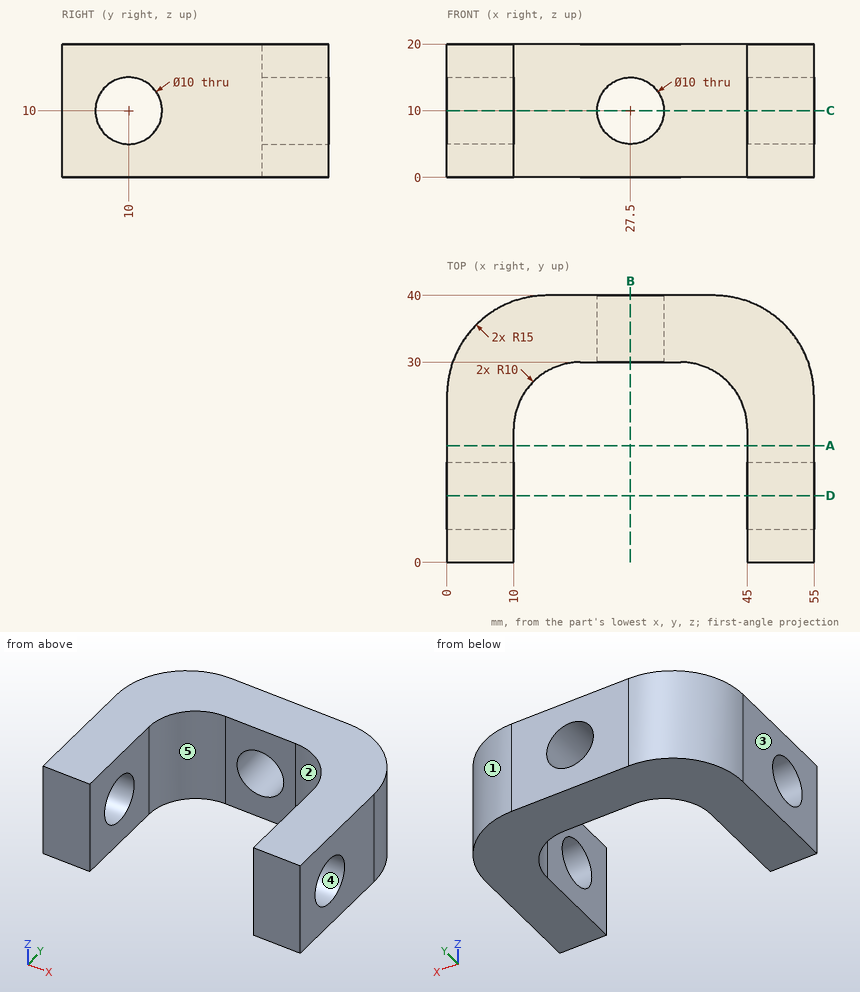
Study the drawing (mm; zero at the part's minimum x, y, z) and answer. A direction names the side the tool comes from. Give positions to 0.01 mm unless a question says otherwise; leave off trailing zeros. Write each loop counter-clockwise with the first axis right and the second up, starting at its lowest first coordinate (ties: lowest second). Pieces come first, ordered by that corner, then holes. Notation, with made-up numbers: (-1.75, 0.25) - (55.25, 0.25) arc R8 cw to (55.25, 15.25) - close; hole circle Ø6 at (33.25, 23.5). An arc over 180 degrees is marked (long way). One line per question, with ' | ' between items. Start each with the question number.
1. Determine the mould class of the marked faces 1, 2 and 3 for opening direction X: +X half, -X half, draft (parallel to the pull), parting line (faces both ways), or undercut.
2. Given P1, Ø4, axis at x = 28.5, z = 5.5, coming from the -Y side; P2, Ø12, axis at x = 24.5, z = 10, coming from the -Y side; P3, Ø10, axis at y = 35, z = 6, coming from the +X side, each flat-ended and moving along its own axis, determine where each tip first touches the part or whether it passes through.
3. Section B-B, the plane x = 27.5 is taken. Determine the outline of the cut face in (y, z), then the cut area to 3 significant figures.
4. Section C-C, the plane z = 10 is taken. Determine the outline of the cut face in (x, y), then the cut area to 3 significant figures.
5. Straight lines are drawn through the part: line 1 (Z direction, x = 27, y = 38); line 2 (X direction, y = 33.5, z = 10); line 3 (Z direction, x = 5, y = 6). For each, find the intervals that lie inside material, in ascending order.
6. Section D-D, the plane y = 10 is taken. Determine the outline of the cut face in (x, z).
7. Section A-A, the plane y = 17.5 is taken. Determine the outline of the cut face in (x, z).
8. For the marked faces 4 and 5, determine the directions among +Z, -Z, +X, -X, +Y, -Y from which every point of the face is accessible in a straight line to the end or side of a thin tool.
Result:
1) face 1: +X half | face 2: undercut | face 3: -X half
2) P1: stops at y = 30 | P2: stops at y = 29.89 | P3: stops at x = 54.14
3) outline: (30, 0) - (40, 0) - (40, 5) - (30, 5) - close; (30, 15) - (40, 15) - (40, 20) - (30, 20) - close | area: 100 mm2
4) outline: (0, 0) - (10, 0) - (10, 5) - (0, 5) - close; (0, 15) - (10, 15) - (10, 20) arc R10 cw to (20, 30) - (22.5, 30) - (22.5, 40) - (15, 40) arc R15 ccw to (0, 25) - close; (32.5, 30) - (35, 30) arc R10 cw to (45, 20) - (45, 15) - (55, 15) - (55, 25) arc R15 ccw to (40, 40) - (32.5, 40) - close; (45, 0) - (55, 0) - (55, 5) - (45, 5) - close | area: 796 mm2
5) line 1: z = 0 to 5.03, 14.97 to 20 | line 2: x = 2.64 to 22.5, 32.5 to 52.36 | line 3: z = 0 to 7, 13 to 20
6) outline: (0, 0) - (10, 0) - (10, 5) - (0, 5) - close; (0, 15) - (10, 15) - (10, 20) - (0, 20) - close; (45, 0) - (55, 0) - (55, 5) - (45, 5) - close; (45, 15) - (55, 15) - (55, 20) - (45, 20) - close
7) outline: (0, 0) - (10, 0) - (10, 20) - (0, 20) - close; (45, 0) - (55, 0) - (55, 20) - (45, 20) - close
8) face 4: +X, -X | face 5: +Z, -Z, -Y
